Check sheet for the modelled part. Datum: model origin and axes. Units: mm. Face numbers are marked on the shaded views. A direction names the side the tool comes from. Give positions to 0.01 mm unless a question says otherwise; leave off trailing zeros. Order: outer loops, then holes, each group sorted by start corner. A loop starts at its lowest first (then second) coordinate and runs counter-clockwise, first axis right, second up. Notation, with made-up numbers: (68.5, 8) -> (119.5, 8) arc R21 cw to (119.5, 29) -> close; hole circle Ø9 at (34, 82). An arc over 180 degrees is marked (long way). Answer in a Markdown table with one row per item. Add a question column.
(1) Cross-section at B-B (z = -127.75). Record the cut outline in (x, y) (3 decimals), then the cut area to 3 significant figures.
(2) Cross-section at A-A (x = 118.25). Record the cut outline in (y, z) (3 decimals).
(3) Cross-section at C-C (x = 128.5). Record the cut outline in (y, z) (3 decimals).
(4) Thickness scan on L1, parallel to Z at x = 108.5, y = 1.8; L2, parallel to X at y = 1.3, z = -128.5; L3, parallel to Z at x = 111.5, y = 2.95. Record the ranges inside material, lowest first. Write a range as [from, to].
(5) Set-up check for the marked faces 1, 2 and 3: record each of +Z, -Z, +X, -X, +Y, -Y from which the full face is reachable in a straight line by a thin tool's end or side.
(6) Release check for a two-part mould opening along Z. For the marked faces 4, 5 and 6 record: released by +Z, released by -Z, zero draft, split by the parting line, or undercut.
(7) Cross-section at D-D (y = 2.6). State how many separate pieces and enclosed holes the cut face has, then the cut area to 3 significant figures.
(8) Go/stop test with flat-tipped pins: pin 1 (1.5 mm diameter, centred on y = 2, z = -113.5, fed in from +X); pin 2 (1.6 mm diameter, centred on x = 108.72, z = -110.47, fed in from +Y); pin 3 (1 mm diameter, centred on x = 129, y = 1.5, fed in from -Z); pin 4 (1 mm diameter, centred on x = 108, y = 2, fed in from +Z). Record where each tip stops, or that it passes through.
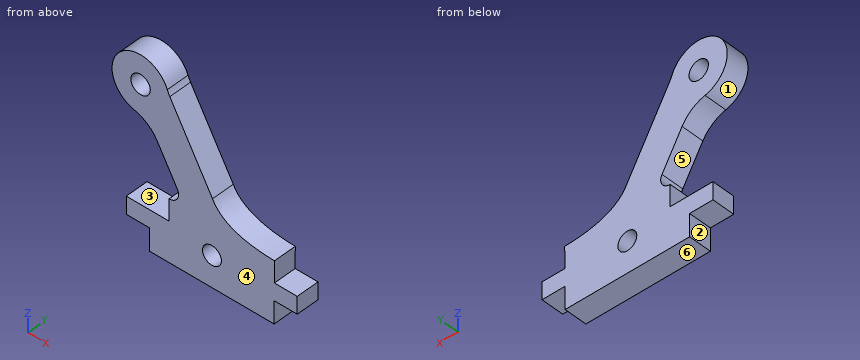
```python
from build123d import *

# Parameters (mm, degrees)
SKETCH1_R           = 1.36
SKETCH1_R_2         = 1.3250121
BOSS_EXTRUDE1_DEPTH = 3.175


with BuildPart() as part:
    # Sketch1 → Boss-Extrude1 (new body)
    with BuildSketch(Plane(origin=(0, 0, 0), x_dir=(1, 0, 0), z_dir=(0, 1, 0))):
        with BuildLine():
            Line((112.722877294, 126.593302228), (112.72277638, 123.593222295))
            ThreePointArc((112.72277638, 123.593222295), (113.875226377, 122.941979767), (113.863024117, 121.61830725))
            Line((113.863024117, 121.61830725), (111.050643934, 116.74721322))
            ThreePointArc((111.050643934, 116.74721322), (109.689478532, 115.224141686), (107.832794667, 114.372529579))
            ThreePointArc((107.832794667, 114.372529579), (105.709889346, 107.841486649), (112.467185669, 109.066311194))
            ThreePointArc((112.467185669, 109.066311194), (112.627253492, 109.444515831), (112.817819601, 109.808308371))
            Line((112.817819601, 109.808308371), (118.803678696, 120.175836459))
            add(Edge.make_bspline(
                [(118.803678696, 120.175836459), (120.361778696, 123.269636459), (125.055778696, 123.618636459), (127.497578696, 123.636436459)],
                knots=[0.666666667, 0.666666667, 0.666666667, 0.666666667, 0.708333333, 0.708333333, 0.708333333, 0.708333333], degree=3))
            Line((127.497578696, 123.636436459), (127.475978696, 126.636436459))
            Line((127.475978696, 126.636436459), (130.675779856, 126.636436459))
            Line((130.675779856, 126.636436459), (130.675779856, 129.036436459))
            Line((130.675779856, 129.036436459), (127.440025111, 129.036436459))
            Line((127.440025111, 129.036436459), (127.440025111, 132.168236459))
            Line((127.440025111, 132.168236459), (109.997615958, 132.168236459))
            Line((109.997615958, 132.168236459), (109.997615958, 129.036436459))
            Line((109.997615958, 129.036436459), (106.722915958, 129.036436459))
            Line((106.722915958, 129.036436459), (106.722915958, 126.593302228))
            Line((106.722915958, 126.593302228), (112.722877294, 126.593302228))
        make_face()
        with Locations(Location((108.72260063, 110.472754541, 0), (0, 0, 270))):
            Circle(SKETCH1_R, mode=Mode.SUBTRACT)
        with Locations(Location((118.723210584, 127.836436459, 0), (0, 0, 270))):
            Circle(SKETCH1_R_2, mode=Mode.SUBTRACT)
    extrude(amount=BOSS_EXTRUDE1_DEPTH)


solid = part.part
```
Answer below:
| question | item | result |
|---|---|---|
| 1 | outline | (106.723, 0) -> (117.401, 0) -> (117.401, 3.175) -> (106.723, 3.175) -> close; (120.045, 0) -> (130.676, 0) -> (130.676, 3.175) -> (120.045, 3.175) -> close |
| 1 | area | 67.7 mm² |
| 2 | outline | (0, -132.168) -> (3.175, -132.168) -> (3.175, -129.074) -> (0, -129.074) -> close; (0, -126.599) -> (3.175, -126.599) -> (3.175, -119.217) -> (0, -119.217) -> close |
| 3 | outline | (0, -129.036) -> (3.175, -129.036) -> (3.175, -126.636) -> (0, -126.636) -> close |
| 4 | L1 | z = [-129.04, -126.59], [-114.57, -111.81], [-109.13, -106.48] |
| 4 | L2 | x = [106.72, 117.58], [119.87, 130.68] |
| 4 | L3 | z = [-132.17, -126.59], [-117.53, -107.59] |
| 5 | face 1 | +Y, -Y |
| 5 | face 2 | -Z, -X, +Y, -Y |
| 5 | face 3 | -X, +Y, -Y |
| 6 | face 4 | zero draft |
| 6 | face 5 | undercut |
| 6 | face 6 | released by -Z |
| 7 | separate pieces | 1 |
| 7 | enclosed holes | 2 |
| 7 | area | 265 mm² |
| 8 | pin 1 | stops at x = 115.38 |
| 8 | pin 2 | passes through |
| 8 | pin 3 | stops at z = -129.04 |
| 8 | pin 4 | stops at z = -106.48 |
